from build123d import *

# Parameters (mm, degrees)
F0_R     = 4.25
F1_DEPTH = 8


with BuildPart() as f1:
    # F0 (on Front) → F1 (new body)
    with BuildSketch(Plane.XZ):
        with BuildLine():
            Line((0, -183.0111), (0, 0))
            Line((0, 0), (0, 15))
            Line((0, 15), (-53, 15))
            ThreePointArc((-53, 15), (-60.071068, 12.071068), (-63, 5))
            Line((-63, 5), (-63, -5))
            ThreePointArc((-63, -5), (-60.071068, -12.071068), (-53, -15))
            Line((-53, -15), (-16, -15))
            ThreePointArc((-16, -15), (-8.928932, -17.928932), (-6, -25))
            Line((-6, -25), (-6, -149))
            ThreePointArc((-6, -149), (-8.928932, -156.071068), (-16, -159))
            Line((-16, -159), (-22.579605, -159))
            Line((-22.579605, -159), (-116, -159))
            ThreePointArc((-116, -159), (-123.071068, -161.928932), (-126, -169))
            Line((-126, -169), (-126, -179))
            ThreePointArc((-126, -179), (-123.071068, -186.071068), (-116, -189))
            Line((-116, -189), (0, -189))
            Line((0, -189), (0, -183.0111))
        make_face()
        with Locations((-111, -174)):
            Circle(F0_R, mode=Mode.SUBTRACT)
        with Locations((-37, -174)):
            Circle(F0_R, mode=Mode.SUBTRACT)
        with Locations((-46, 0)):
            Circle(F0_R, mode=Mode.SUBTRACT)
    extrude(amount=F1_DEPTH)


solid = f1.part
Input: part model. Units: mm. Frame: model coordinates. A direction names the side the tool comes from. Round coordinates to 2 decimals unless told otherwise and drop trailing zeros. Order: outer loops, then holes, each group sorted by start corner. A loop starts at its lowest first (then second) coordinate and runs counter-clockwise, first axis right, second up. Notation, with made-up numbers: (-22, 85.25) - (-5, 85.25) arc R36 cw to (-5, 120.25) - close; hole circle Ø7 at (19, -5.75). An arc over 180 degrees is marked (long way). Answer as a JSON object with one key per item and string values. Group by question number.
(1) Pin query (flat end, axial travel): P1, Ø7.5, axis at x = -46, z = 0, coming from the +Y side; P2, Ø2.5, axis at y = -2.5, z = -86.5, coming from the -X side; P3, Ø11, axis at x = -111, z = -174, coming from the -Y side; P4, Ø4, axis at x = -90, y = -5, coming from the +Z side. Return the tip coordinate at first contact, or that it passes through.
(2) Cut plane D-D (x = -46). Return loops of the section in (y, z), then the cut area to 3 significant figures.
(3) Cut plane B-B (x = -111). Return loops of the section in (y, z).
(4) Cut plane A-A (z = -174). Return loops of the section in (x, y), then the cut area to 3 significant figures.
(5) Cut plane C-C (y = -3.5). Return loops of the section in (x, z), then the cut area to 3 significant figures.
(6) Draft query along X for faces 4 (the face through (-65, -4, -159)), 5 (the face through (-122.99, -3.94, -161.85)), 6 (the face through (0, -4, -88)), 7 (the face through (-40.132, -3.944, -171.128)). Return one class per face: released by +X, released by -X, zero draft, split by the parting line, or undercut.
(7) Reachability of faces 1 (the face through (-9.01, -3.94, -17.85)), 2 (the face through (-63, -4, 0)), 3 (the face through (-115.246, -3.944, -173.813)) from +Z, -Z, +X, -X, +Y, -Y: full face, straight path, thin tool, end or side. Return the list, or none.
(8) Material intervals for probe 1 along Z at (x, y) = (-46, -5.25); probe 2 along Z at (x, y) = (-111, -3.25); probe 3 along Z at (x, y) = (-40, -1), sorted ascending. Write a range as from..to.
Here are the results:
{
 "1": {"P1": "passes through", "P2": "stops at x = -6", "P3": "stops at y = -8", "P4": "stops at z = -159"},
 "2": {"outline": "(-8, -189) - (0, -189) - (0, -159) - (-8, -159) - close; (-8, -15) - (0, -15) - (0, -4.25) - (-8, -4.25) - close; (-8, 4.25) - (0, 4.25) - (0, 15) - (-8, 15) - close", "area": "412 mm^2"},
 "3": {"outline": "(-8, -189) - (0, -189) - (0, -178.25) - (-8, -178.25) - close; (-8, -169.75) - (0, -169.75) - (0, -159) - (-8, -159) - close"},
 "4": {"outline": "(-126, -8) - (-115.25, -8) - (-115.25, 0) - (-126, 0) - close; (-106.75, -8) - (-41.25, -8) - (-41.25, 0) - (-106.75, 0) - close; (-32.75, -8) - (0, -8) - (0, 0) - (-32.75, 0) - close", "area": "872 mm^2"},
 "5": {"outline": "(-126, -179) arc R10 ccw to (-116, -189) - (0, -189) - (0, 15) - (-53, 15) arc R10 ccw to (-63, 5) - (-63, -5) arc R10 ccw to (-53, -15) - (-16, -15) arc R10 cw to (-6, -25) - (-6, -149) arc R10 cw to (-16, -159) - (-116, -159) arc R10 ccw to (-126, -169) - close; hole circle Ø8.5 at (-111, -174); hole circle Ø8.5 at (-46, 0); hole circle Ø8.5 at (-37, -174)", "area": "6,320 mm^2"},
 "6": {"face 4": "zero draft", "face 5": "released by -X", "face 6": "released by +X", "face 7": "undercut"},
 "7": {"face 1": "-X, +Y, -Y", "face 2": "+Z, -X, +Y, -Y", "face 3": "+Y, -Y"},
 "8": {"probe 1": "z = -189..-159, -15..-4.25, 4.25..15", "probe 2": "z = -189..-178.25, -169.75..-159", "probe 3": "z = -189..-177.01, -170.99..-159, -15..15"}
}
